```python
from build123d import *

# Parameters (mm, degrees)
SKETCH_1_R                   = 48
EXTRUDE_1_DEPTH              = 5
HOLE_WIZARD_M3_1_AT_2_COUNT  = 2
HOLE_WIZARD_M3_1_AT_2_PITCH  = 12
HOLE_WIZARD_M3_1_AT_3_COUNT  = 2
HOLE_WIZARD_M3_1_AT_3_PITCH  = 24
HOLE_WIZARD_M3_1_AT_4_COUNT  = 2
HOLE_WIZARD_M3_1_AT_4_PITCH  = 36
HOLE_WIZARD_M3_1_AT_5_COUNT  = 2
HOLE_WIZARD_M3_1_AT_5_PITCH  = 48
HOLE_WIZARD_M3_1_AT_6_COUNT  = 2
HOLE_WIZARD_M3_1_AT_6_PITCH  = 59
HOLE_WIZARD_M3_1_AT_7_COUNT  = 2
HOLE_WIZARD_M3_1_AT_7_PITCH  = 60.207972894
HOLE_WIZARD_M3_1_AT_8_COUNT  = 2
HOLE_WIZARD_M3_1_AT_8_PITCH  = 63.694583757
HOLE_WIZARD_M3_1_AT_9_COUNT  = 2
HOLE_WIZARD_M3_1_AT_9_PITCH  = 69.115844783
HOLE_WIZARD_M3_1_AT_10_COUNT = 2
HOLE_WIZARD_M3_1_AT_10_PITCH = 76.059187479
CUT_EXTRUDE_1_REACH          = 70.066
SKETCH_5_R                   = 2
PATTERN_CIRCULAR_1_COUNT     = 6


with BuildPart() as part:
    # 草圖1 → 填料-伸長1 (new body)
    with BuildSketch(Plane.XY):
        Circle(SKETCH_1_R)
    extrude(amount=EXTRUDE_1_DEPTH)

    # 草圖4 → M3 六角承窩頭蓋螺釘的柱孔1 (revolve, cut)
    with BuildSketch(Plane(origin=(-29.5, 24, 0), x_dir=(0, 1, 0), z_dir=(1, 0, 0))):
        Polygon((0, 0), (0, 5), (1.7, 5), (1.7, 3.4), (3.25, 3.4), (3.25, 0.025), (3.275, 0), align=None)
    hole_wizard_m3_1 = revolve(axis=Axis((-29.5, 24, -6.35), (0, 0, 1)), mode=Mode.SUBTRACT)

    # M3 六角承窩頭蓋螺釘的柱孔1 at 2: M3 六角承窩頭蓋螺釘的柱孔1 ×2
    with Locations(*[(0, -i * HOLE_WIZARD_M3_1_AT_2_PITCH, 0) for i in range(1, HOLE_WIZARD_M3_1_AT_2_COUNT)]):
        add(hole_wizard_m3_1, mode=Mode.SUBTRACT)

    # M3 六角承窩頭蓋螺釘的柱孔1 at 3: M3 六角承窩頭蓋螺釘的柱孔1 ×2
    with Locations(*[(0, -i * HOLE_WIZARD_M3_1_AT_3_PITCH, 0) for i in range(1, HOLE_WIZARD_M3_1_AT_3_COUNT)]):
        add(hole_wizard_m3_1, mode=Mode.SUBTRACT)

    # M3 六角承窩頭蓋螺釘的柱孔1 at 4: M3 六角承窩頭蓋螺釘的柱孔1 ×2
    with Locations(*[(0, -i * HOLE_WIZARD_M3_1_AT_4_PITCH, 0) for i in range(1, HOLE_WIZARD_M3_1_AT_4_COUNT)]):
        add(hole_wizard_m3_1, mode=Mode.SUBTRACT)

    # M3 六角承窩頭蓋螺釘的柱孔1 at 5: M3 六角承窩頭蓋螺釘的柱孔1 ×2
    with Locations(*[(0, -i * HOLE_WIZARD_M3_1_AT_5_PITCH, 0) for i in range(1, HOLE_WIZARD_M3_1_AT_5_COUNT)]):
        add(hole_wizard_m3_1, mode=Mode.SUBTRACT)

    # M3 六角承窩頭蓋螺釘的柱孔1 at 6: M3 六角承窩頭蓋螺釘的柱孔1 ×2
    with Locations(*[(i * HOLE_WIZARD_M3_1_AT_6_PITCH, 0, 0) for i in range(1, HOLE_WIZARD_M3_1_AT_6_COUNT)]):
        add(hole_wizard_m3_1, mode=Mode.SUBTRACT)

    # M3 六角承窩頭蓋螺釘的柱孔1 at 7: M3 六角承窩頭蓋螺釘的柱孔1 ×2
    with Locations(*[Vector(0.9799366622741338, -0.19930915164896565, 0) * (i * HOLE_WIZARD_M3_1_AT_7_PITCH) for i in range(1, HOLE_WIZARD_M3_1_AT_7_COUNT)]):
        add(hole_wizard_m3_1, mode=Mode.SUBTRACT)

    # M3 六角承窩頭蓋螺釘的柱孔1 at 8: M3 六角承窩頭蓋螺釘的柱孔1 ×2
    with Locations(*[Vector(0.9262954009547517, -0.37679812920193184, 0) * (i * HOLE_WIZARD_M3_1_AT_8_PITCH) for i in range(1, HOLE_WIZARD_M3_1_AT_8_COUNT)]):
        add(hole_wizard_m3_1, mode=Mode.SUBTRACT)

    # M3 六角承窩頭蓋螺釘的柱孔1 at 9: M3 六角承窩頭蓋螺釘的柱孔1 ×2
    with Locations(*[Vector(0.8536392803366317, -0.5208646456291284, 0) * (i * HOLE_WIZARD_M3_1_AT_9_PITCH) for i in range(1, HOLE_WIZARD_M3_1_AT_9_COUNT)]):
        add(hole_wizard_m3_1, mode=Mode.SUBTRACT)

    # M3 六角承窩頭蓋螺釘的柱孔1 at 10: M3 六角承窩頭蓋螺釘的柱孔1 ×2
    with Locations(*[Vector(0.7757116786991063, -0.6310874674162169, 0) * (i * HOLE_WIZARD_M3_1_AT_10_PITCH) for i in range(1, HOLE_WIZARD_M3_1_AT_10_COUNT)]):
        add(hole_wizard_m3_1, mode=Mode.SUBTRACT)

    # 草圖5 → 除料-伸長1 (cut, up to next)
    with BuildSketch(Plane(origin=(0, 0, 0), x_dir=(-1, 0, 0), z_dir=(0, 0, -1)), mode=Mode.PRIVATE) as cut_extrude_1_sk1:
        with Locations((0, 15.5)):
            Circle(SKETCH_5_R)
    cut_extrude_1_tool1 = extrude(cut_extrude_1_sk1.sketch, amount=-CUT_EXTRUDE_1_REACH, mode=Mode.PRIVATE) & part.part
    cut_extrude_1 = cut_extrude_1_tool1.solids().sort_by_distance((0, 15.5, 0))[0]
    add(cut_extrude_1, mode=Mode.SUBTRACT)

    # 環狀複製排列1: 除料-伸長1 ×6 about axis
    pattern_circular_1_axis = Axis((0, 0, 0), (0, 0, 1))
    for i in range(1, PATTERN_CIRCULAR_1_COUNT):
        add(cut_extrude_1.rotate(pattern_circular_1_axis, i * 360 / PATTERN_CIRCULAR_1_COUNT), mode=Mode.SUBTRACT)


solid = part.part
```
Work out the finished part from the listing and answer in its coordinate system (mm). A direction names the side the tool comes from. Round coordinates to 2 decimals unless told otherwise and drop trailing zeros. Order: outer loops, then holes, each group sorted by start corner. A loop starts at its lowest first (then second) coordinate and runs counter-clockwise, first axis right, second up.
Q1. The mould has two halves that part along X. Classify faces 3 (the cylindrical face through (32.383, -22.5, 1.689)), 4 (the flat face through (-1, 1, 5)): pulls with the +X half, pulls with the -X half, needs draft (parallel to the pull), parting line crosses it, or undercut.
Solution:
face 3: undercut
face 4: needs draft
Q2. Find the intervals of material crossed by line 1 along X through (y, z) = (-2, 0.75); line 2 along Y through (x, z) = (-29.5, 1.8); line 3 along Y through (x, z) = (29, 0.25), in increasing order.
Solution:
line 1: x = -47.96 to -32.06, -26.94 to 26.94, 32.06 to 47.96
line 2: y = -37.86 to -27.25, -20.75 to -15.25, -8.75 to -3.25, 3.25 to 8.75, 15.25 to 20.75, 27.25 to 37.86
line 3: y = -38.25 to -27.21, -20.79 to -15.21, -8.79 to -3.21, 3.21 to 8.79, 15.21 to 20.79, 27.21 to 38.25
Q3. A cutting plane is placed at C-C, the plane y = 12. Determine the outline of the cut face in (x, z) (3 decimals).
Solution:
outline: (-46.476, 0) - (-32.775, 0) - (-32.75, 0.025) - (-32.75, 3.4) - (-31.2, 3.4) - (-31.2, 5) - (-46.476, 5) - close; (-27.8, 3.4) - (-26.25, 3.4) - (-26.25, 0.025) - (-26.225, 0) - (26.225, 0) - (26.25, 0.025) - (26.25, 3.4) - (27.8, 3.4) - (27.8, 5) - (-27.8, 5) - close; (31.2, 3.4) - (32.75, 3.4) - (32.75, 0.025) - (32.775, 0) - (46.476, 0) - (46.476, 5) - (31.2, 5) - close
Q4. Given pin 1 Ø1.5 at (y, z) = (22.5, 3.5) entering from -X; pin 2 Ø2.5 at (x, y) = (-29.5, -24) entering from +Z; pin 3 Ø2 at (y, z) = (-26, 3.5) entering from +X; pin 4 Ø4.5 at (x, y) = (29.5, 0) entering from -Z, each flat-ended and moving along its own axis, determine where each tip first touches the part or whether it passes through.
Solution:
pin 1: stops at x = -42.79
pin 2: passes through
pin 3: stops at x = 40.98
pin 4: stops at z = 3.4
Q5. A tool of negligible diameter and unlimited length cuts with its end or side. For faces 1 (the cylindrical face through (-28.85, -10.43, 4.19)), 2 (the cylindrical face through (-26.327, -24.705, 1.689)), from which of +Z, -Z, +X, -X, +Y, -Y can it reach the whole face along a straight path? Write none if from no direction.
Solution:
face 1: +Z, -Z
face 2: -Z
Q6. A cutting plane is placed at B-B, the plane z = 1.7. Count the separate pieces of the cut face and the enclosed holes in it, then the cut area to 3 significant figures.
Solution:
separate pieces: 1
enclosed holes: 16
area: 6,830 mm2
Q7. A cutting plane is placed at A-A, the plane y = 0. Determine the outline of the cut face in (x, z) (3 decimals).
Solution:
outline: (-48, 0) - (-32.775, 0) - (-32.75, 0.025) - (-32.75, 3.4) - (-31.2, 3.4) - (-31.2, 5) - (-48, 5) - close; (-27.8, 3.4) - (-26.25, 3.4) - (-26.25, 0.025) - (-26.225, 0) - (26.225, 0) - (26.25, 0.025) - (26.25, 3.4) - (27.8, 3.4) - (27.8, 5) - (-27.8, 5) - close; (31.2, 3.4) - (32.75, 3.4) - (32.75, 0.025) - (32.775, 0) - (48, 0) - (48, 5) - (31.2, 5) - close
